Work out the finished part from the listing and answer in its coordinate system (mm). Face numbers are marked on the shaded views. A direction names the side the tool comes from. Coordinates: 2 decimals unless noted, no trailing zeros. Loops run counter-clockwise (first coordinate to the right, second up) from the corner with the lowest first, then second, coordinate; pieces in that order, holes last.
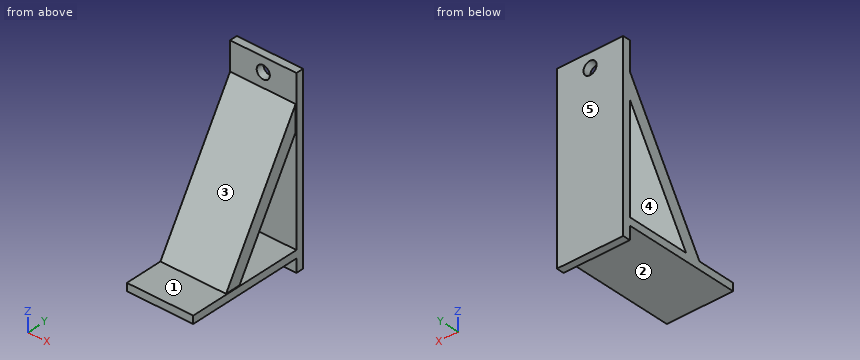
```python
from build123d import *

# Parameters (mm, degrees)
F0_W     = 25.31
F0_H     = 69
F1_DEPTH = 1.45
F2_W     = 25.31
F2_H     = 2.9
F3_DEPTH = 44.64
F8_DEPTH = 25
F10_D    = 5


with BuildPart() as f1:
    # F0 (on Front) → F1 (new body, symmetric)
    with BuildSketch(Plane.XZ):
        Rectangle(F0_W, F0_H)
    extrude(amount=F1_DEPTH, both=True)

    # F2 (on face) → F3 (join)
    with BuildSketch(Plane.XZ.offset(1.45)):
        with Locations((0, -28.05)):
            Rectangle(F2_W, F2_H)
    extrude(amount=F3_DEPTH)

    # F7 (on line) → F8 (join)
    with BuildSketch(Plane(origin=(-12.655, 0, 0), x_dir=(0, -1, 0), z_dir=(-1, 0, 0))):
        Polygon((25.722218447, -26.6), (31.55, -26.6), (1.45, 23.67), (1.45, 13.9370239645), align=None)
    extrude(amount=-F8_DEPTH)

    # F10 (through all)
    with Locations(Plane.XZ.offset(1.45)):
        with Locations((0, 29.1)):
            Hole(F10_D / 2)


solid = f1.part
```
1. A cutting plane is placed at C-C, the plane x = -9. Give the vertices of the cut face in (y, z).
2. A cutting plane is placed at D-D, the plane y = -14. Give the vertices of the cut face in (x, z) (3 decimals).
3. A cutting plane is placed at B-B, the plane z = 29.1. Give the vertices of the cut face in (x, y) (3 decimals).
4. Determine the mould class of the marked faces 1, 2 and 3 for opening direction Z: released by +Z, released by -Z, zero draft, split by the parting line, or undercut.
5. For the marked faces 4 and 5, determine the directions among +Z, -Z, +X, -X, +Y, -Y from which every point of the face is accessible in a straight line to the end or side of a thin tool.
6. Each of these flat-tipped pins is pushed along its axis until it touches: P1, Ø5, axis at x = -0.5, z = -18, coming from the -Y side; P2, Ø12, axis at x = -3, y = -25, coming from the +Z side; P3, Ø6, axis at x = -3, y = -35.5, coming from the +Z side; P4, Ø8, axis at y = -8, z = -16, coming from the +X side. Where does it stop, or does it pass through?
7. Straight lines are drawn through the part: probe 1 along X at (y, z) = (0, 29) (3 decimals); probe 2 along Z at (x, y) = (0, 0.8); probe 3 along Y at (x, z) = (-9.25, 28). For each, find the intervals that lie inside material, in ascending order.
8. A cutting plane is placed at A-A, the plane x = 0. Give the vertices of the cut face in (y, z).
Answers below:
1. outline: (-46.09, -29.5) - (-1.45, -29.5) - (-1.45, -34.5) - (1.45, -34.5) - (1.45, 34.5) - (-1.45, 34.5) - (-1.45, 23.67) - (-31.55, -26.6) - (-46.09, -26.6) - close; hole (-25.72, -26.6) - (-1.45, -26.6) - (-1.45, 13.94) - close
2. outline: (-12.655, -29.5) - (12.655, -29.5) - (12.655, -26.6) - (-12.655, -26.6) - close; (-12.655, -7.023) - (12.345, -7.023) - (12.345, 2.71) - (-12.655, 2.71) - close
3. outline: (-12.655, -1.45) - (-2.5, -1.45) - (-2.5, 1.45) - (-12.655, 1.45) - close; (2.5, -1.45) - (12.655, -1.45) - (12.655, 1.45) - (2.5, 1.45) - close
4. face 1: undercut
4. face 2: released by -Z
4. face 3: released by +Z
5. face 4: +X, -X
5. face 5: +Z, -Z, +X, -X, +Y
6. P1: stops at y = -27.9
6. P2: stops at z = -5.64
6. P3: stops at z = -26.6
6. P4: passes through
7. probe 1: x = -12.655 to -2.498, 2.498 to 12.655
7. probe 2: z = -34.5 to 26.6, 31.6 to 34.5
7. probe 3: y = -1.45 to 1.45
8. outline: (-46.09, -29.5) - (-1.45, -29.5) - (-1.45, -34.5) - (1.45, -34.5) - (1.45, 26.6) - (-1.45, 26.6) - (-1.45, 23.67) - (-31.55, -26.6) - (-46.09, -26.6) - close; (-1.45, 31.6) - (1.45, 31.6) - (1.45, 34.5) - (-1.45, 34.5) - close; hole (-25.72, -26.6) - (-1.45, -26.6) - (-1.45, 13.94) - close
